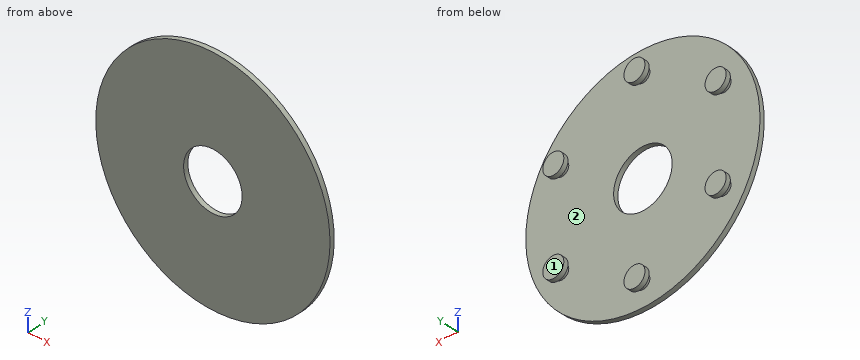
from build123d import *

# Parameters (mm, degrees)
SKETCH1_R           = 50
BOSS_EXTRUDE1_DEPTH = 2
SKETCH2_R           = 12.5
CUT_EXTRUDE1_DEPTH  = 2
SKETCH2_3_R         = 4.5
BOSS_EXTRUDE2_DEPTH = 4
SKETCH2_4_R         = 4.5
SKETCH2_4_R_2       = 3
CUT_EXTRUDE2_DEPTH  = 2
CIRPATTERN1_COUNT   = 12


with BuildPart() as part:
    # Sketch1 → Boss-Extrude1 (new body)
    with BuildSketch(Plane(origin=(0, 0, 0), x_dir=(1, 0, 0), z_dir=(0, 1, 0))):
        with Locations(Location((0, 0, 0), (0, 0, 270))):
            Circle(SKETCH1_R)
    extrude(amount=BOSS_EXTRUDE1_DEPTH)

    # Sketch2 → Cut-Extrude1 (cut)
    with BuildSketch(Plane(origin=(0, 2, 0), x_dir=(1, 0, 0), z_dir=(0, 1, 0))):
        with Locations(Location((0, 0, 0), (0, 0, 270))):
            Circle(SKETCH2_R)
    extrude(amount=-CUT_EXTRUDE1_DEPTH, mode=Mode.SUBTRACT)

    # Sketch2<3> → Boss-Extrude2 (add)
    with BuildSketch(Plane(origin=(0, 2, 0), x_dir=(1, 0, 0), z_dir=(0, 1, 0))):
        with Locations(Location((0, -40, 0), (0, 0, 270))):
            Circle(SKETCH2_3_R)
    boss_extrude2 = extrude(amount=BOSS_EXTRUDE2_DEPTH)

    # Sketch2<4> → Cut-Extrude2 (cut)
    with BuildSketch(Plane(origin=(0, 2, 0), x_dir=(1, 0, 0), z_dir=(0, 1, 0))):
        with Locations(Location((0, -40, 0), (0, 0, 270))):
            Circle(SKETCH2_4_R)
        with Locations(Location((0, -40, 0), (0, 0, 270))):
            Circle(SKETCH2_4_R_2, mode=Mode.SUBTRACT)
    cut_extrude2 = extrude(amount=CUT_EXTRUDE2_DEPTH, mode=Mode.SUBTRACT)

    # CirPattern1: Boss-Extrude2, Cut-Extrude2 ×12 about axis, 6 skipped
    cirpattern1_axis = Axis((0, -35.355339059, 0), (0, 1, 0))
    add([boss_extrude2.rotate(cirpattern1_axis, i * 360 / CIRPATTERN1_COUNT) for i in range(1, CIRPATTERN1_COUNT) if i not in (1, 3, 5, 7, 9, 11)])
    add([cut_extrude2.rotate(cirpattern1_axis, i * 360 / CIRPATTERN1_COUNT) for i in range(1, CIRPATTERN1_COUNT) if i not in (1, 3, 5, 7, 9, 11)], mode=Mode.SUBTRACT)


solid = part.part
Here's how the part is built. I have some questions about the finished solid (model axes, mm). Face numbers are marked on the shaded views. Give positions to 0.01 mm unless a question says otherwise; leave off trailing zeros. Loops run counter-clockwise (first coordinate to the right, second up) from the corner with the lowest first, then second, coordinate; pieces in that order, holes last. Notation, with made-up numbers: (87.25, 46) -> (136.25, 46) arc R8 cw to (136.25, 55) -> close; hole circle Ø1 at (30.5, -40). An arc over 180 degrees is marked (long way). Answer as a JSON object with one key per item and string values. Group by question number.
Item 1: Will these pins go through, and if not, where does the flat tip stop? pin 1 (10 mm diameter, centred on x = -15, z = 7, fed in from +Y); pin 2 (1.5 mm diameter, centred on y = 3.5, z = 19.5, fed in from +X).
Item 2: I need wall thicknesses on L1, parallel to X at y = 0.6, z = 0; L2, parallel to Y at x = 15.5, z = 5; L3, parallel to X at y = 0.45, z = -8.5. Which ranges of each line are inside material? Lowest first, please.
Item 3: Imagine slicing it at D-D on z = 40. Write out the boundary of the cut face in (x, y), then the cut area to 3 significant figures.
Item 4: Imagine slicing it at A-A on x = 0. Write out the boundary of the cut face in (y, z), then the cut area to 3 significant figures.
Item 5: Imagine slicing it at B-B on z = 0. Write out the boundary of the cut face in (x, y).
Item 6: Thinking about a two-plate mould opening in X: for the marked faces 1 and 2, which applies, pulls with the +X half, pulls with the -X half, needs draft (parallel to the pull), parting line crosses it, or undercut?
Item 7: Imagine slicing it at C-C on y = 3.05. Write out the boundary of the cut face in (x, z), then the cut area to 3 significant figures.
Answer list:
{
 "1": {"pin 1": "stops at y = 2", "pin 2": "stops at x = 39.14"},
 "2": {"L1": "x = -50 to -12.5, 12.5 to 50", "L2": "y = 0 to 2", "L3": "x = -49.27 to -9.17, 9.17 to 49.27"},
 "3": {"outline": "(-30, 0) -> (30, 0) -> (30, 2) -> (3, 2) -> (3, 4) -> (4.5, 4) -> (4.5, 6) -> (-4.5, 6) -> (-4.5, 4) -> (-3, 4) -> (-3, 2) -> (-30, 2) -> close", "area": "150 mm2"},
 "4": {"outline": "(0, -50) -> (2, -50) -> (2, -43) -> (4, -43) -> (4, -44.5) -> (6, -44.5) -> (6, -35.5) -> (4, -35.5) -> (4, -37) -> (2, -37) -> (2, -12.5) -> (0, -12.5) -> close; (0, 12.5) -> (2, 12.5) -> (2, 37) -> (4, 37) -> (4, 35.5) -> (6, 35.5) -> (6, 44.5) -> (4, 44.5) -> (4, 43) -> (2, 43) -> (2, 50) -> (0, 50) -> close", "area": "210 mm2"},
 "5": {"outline": "(-50, 0) -> (-12.5, 0) -> (-12.5, 2) -> (-50, 2) -> close; (12.5, 0) -> (50, 0) -> (50, 2) -> (12.5, 2) -> close"},
 "6": {"face 1": "needs draft", "face 2": "undercut"},
 "7": {"outline": "circle Ø6 at (-34.64, -20); circle Ø6 at (-34.64, 20); circle Ø6 at (0, -40); circle Ø6 at (0, 40); circle Ø6 at (34.64, -20); circle Ø6 at (34.64, 20)", "area": "170 mm2"}
}
